Check sheet for the modelled part. Datum: model origin and axes. Units: mm. A direction names the side the tool comes from. Give positions to 0.01 mm unless a question says otherwise; leave off trailing zeros. Write each loop counter-clockwise with the first axis right and the second up, starting at its lowest first coordinate (ties: lowest second). Pieces come first, ordered by that corner, then holes. Notation, with made-up numbers: M -9,61.25 L 17,61.25 A24 ccw 17,77.25 Z; hole C 25,55.5 d10. An arc over 180 degrees is marked long. Write item = value, one per line. Start each with the question number.
1) Sectioned sample at A-A, the plane x = 0. Record the cut outline in (y, z) (3 decimals).
2) Gauge pin test, flat ends, axial feed: pin 1 (2 mm diameter, centred on y = 5.5, z = -2.5, fed in from -X); pin 2 (1 mm diameter, centred on y = 4, z = -1.5, fed in from +X). Record the tip position at first contact, or that the pin passes through.
3) Set-up check for faces 1 (the face through (-1, 5.74, 3)), 2 (the face through (3.233, 0.602, 1.341)): record each of +Z, -Z, +X, -X, +Y, -Y from which the full face is reachable in a straight line by a thin tool's end or side.
4) Scan lines: L1, parallel to Y at x = -1.75, z = 2.5; L2, parallel to Z at x = 0, y = 6 (3 decimals); L3, parallel to X at y = 4.25, z = 1.5. Record each from-to range of solid material in increasing order.
5) Draft check along Y on faces 3 (the face through (-2.2, 6.1, -2)), 4 (the face through (3.233, 8.037, 1.341)), 5 (the face through (2, 9.501, 2)). Enter one of: pulls with the +Y half, pulls with the -Y half, needs draft (parallel to the pull), parting line crosses it, or undercut.
from build123d import *

# Parameters (mm, degrees)
CUT_EXTRUDE1_REACH = 12.713
SKETCH3_R          = 2.067


with BuildPart() as part:
    # Sketch2 → Revolve1 (revolve)
    with BuildSketch(Plane.XY):
        Polygon((0, 0), (3.5, 0), (3.5, 1.188), (2.975, 1.188), (2.975, 2.771), (3.5, 2.771), (3.5, 5.74), (2.975, 5.74), (2.975, 6.532), (3.5, 6.532), (3.5, 9.501), (0, 9.501), align=None)
    revolve(axis=Axis((0, -157.439431358, 0), (0, 1, 0)))

    # Sketch3 → Cut-Extrude1 (cut, up to next)
    with BuildSketch(Plane(origin=(0, 9.501, 0), x_dir=(1, 0, 0), z_dir=(0, 1, 0)), mode=Mode.PRIVATE) as cut_extrude1_sk1:
        with Locations(Location((0, 0, 0), (0, 0, 180))):
            Circle(SKETCH3_R)
    cut_extrude1_tool1 = extrude(cut_extrude1_sk1.sketch, amount=-CUT_EXTRUDE1_REACH, mode=Mode.PRIVATE) & part.part
    add(cut_extrude1_tool1.solids().sort_by_distance((0, 9.501, 0))[0], mode=Mode.SUBTRACT)

    # Sketch14 → Cut-Revolve1 (revolve, cut)
    with BuildSketch(Plane.XY, mode=Mode.PRIVATE) as cut_revolve1_sk:
        Polygon((-2.5, 9.501), (-2.067, 9.068), (-2.067, 9.501), align=None)
        Polygon((-2.5, 0), (-2.067, 0.433), (-2.067, 0), align=None)
    revolve(cut_revolve1_sk.sketch.rotate(Axis((0, -1000, 0), (0, 1, 0)), 180), axis=Axis((0, -1000, 0), (0, 1, 0)), mode=Mode.SUBTRACT)


solid = part.part
Data:
q1.outline = M 0,-3.5 L 1.188,-3.5 L 1.188,-2.975 L 2.771,-2.975 L 2.771,-3.5 L 5.74,-3.5 L 5.74,-2.975 L 6.532,-2.975 L 6.532,-3.5 L 9.501,-3.5 L 9.501,-2.5 L 9.068,-2.067 L 0.433,-2.067 L 0,-2.5 Z; M 0,2.5 L 0.433,2.067 L 9.068,2.067 L 9.501,2.5 L 9.501,3.5 L 6.532,3.5 L 6.532,2.975 L 5.74,2.975 L 5.74,3.5 L 2.771,3.5 L 2.771,2.975 L 1.188,2.975 L 1.188,3.5 L 0,3.5 Z
q2.pin_1 = -3.16
q2.pin_2 = 3.35
q3.face_1 = none
q3.face_2 = +Y, -Y
q4.L1 = 0 to 1.19, 2.77 to 5.74, 6.53 to 9.5
q4.L2 = -2.975 to -2.067, 2.067 to 2.975
q4.L3 = -3.16 to -1.42, 1.42 to 3.16
q5.face_3 = undercut
q5.face_4 = needs draft
q5.face_5 = pulls with the +Y half
